Could you check a few things on this model? Use its own coordinates, in mm. Face numbers are marked on the shaded views. A direction names the side the tool comes from. Round coordinates to 2 decimals unless told otherwise and drop trailing zeros. Write each loop counter-clockwise with the first axis right and the second up, starting at its lowest first coordinate (ties: lowest second). Pieces come first, ordered by that corner, then holes. Notation, with made-up numbers: (-39.75, 43) -> (4.25, 43) arc R18 cw to (4.25, 62) -> close; hole circle Ø3 at (38, 60). An arc over 180 degrees is marked (long way). One line per question, with ' | ' between items. Start each with the question number.
1. If I drill on line 1 along Z through (x, y) = (126.5, -103); line 2 along X through (y, z) = (-125.5, 22.5); line 3 along X through (y, z) = (-34, 20), over which ranges is the centre line in solid material (lowest first)? Write a range as [from, to].
2. For pin 1 Ø5 at (x, y) = (115, -138) entering from -Z; pin 2 Ø3 at (y, z) = (-75, 20.5) entering from +X; pin 3 Ø5 at (x, z) = (75, 17.5) entering from +Y, each with a flat end and sliding along its axis, tell me the tip position at first contact or that it passes through.
3. Imagine slicing it at A-A, the plane x = 21. List the corners of the cut face in (y, z) for me.
4. Imagine slicing it at C-C, the plane y = -73. List the corners of the cut face in (x, z) for me.
5. For the marked faces 1 and 2, which set-ups out of +Z, -Z, +X, -X, +Y, -Y let a thin tool reach every point of the face, with its end or its side?
6. Imagine slicing it at B-B, the plane z = 20.75. List the corners of the cut face in (x, y) for me.
7. Imagine slicing it at D-D, the plane y = -145. List the corners of the cut face in (x, z) for me, and give its area (3 significant figures).
from build123d import *

# Parameters (mm, degrees)
REVOLUTION_ANGLE = -90


with BuildPart() as part:
    # Sketch → Revolution (revolve)
    with BuildSketch(Plane.XZ):
        Polygon((140, 25.020922), (136, 25.020922), (136, 16.020922), (140, 16.020922), (140, 23.020922), (190, 23.020922), (190, 25.020922), align=None)
    revolve(axis=Axis((0, 0, 0), (0, 0, 1)), revolution_arc=REVOLUTION_ANGLE)


solid = part.part
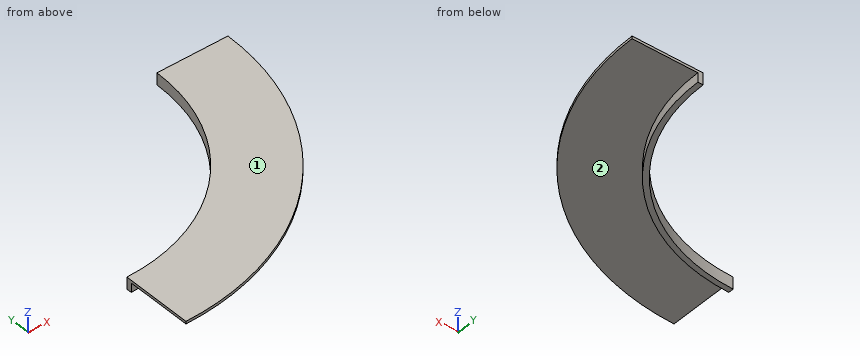
Geometry results:
1) line 1: z = [23.02, 25.02] | line 2: x = [52.4, 62.05] | line 3: x = [131.68, 135.81]
2) pin 1: stops at z = 23.02 | pin 2: stops at x = 119.15 | pin 3: stops at y = -111.76
3) outline: (-188.84, 23.02) -> (-138.42, 23.02) -> (-138.42, 16.02) -> (-134.37, 16.02) -> (-134.37, 25.02) -> (-188.84, 25.02) -> close
4) outline: (114.75, 16.02) -> (119.46, 16.02) -> (119.46, 23.02) -> (175.42, 23.02) -> (175.42, 25.02) -> (114.75, 25.02) -> close
5) face 1: +Z, +X, -X, +Y, -Y | face 2: -Z, +X, -Y
6) outline: (0, -140) arc R140 ccw to (140, 0) -> (136, 0) arc R136 cw to (0, -136) -> close
7) outline: (0, 23.02) -> (122.78, 23.02) -> (122.78, 25.02) -> (0, 25.02) -> close | area: 246 mm2
